Here's how the part is built. I have some questions about the finished solid (model axes, mm). A direction names the side the tool comes from. Coordinates: 2 decimals unless noted, no trailing zeros. Order: outer loops, then holes, each group sorted by start corner. A loop starts at its lowest first (then second) coordinate and runs counter-clockwise, first axis right, second up.
```python
from build123d import *

# Parameters (mm, degrees)
F0_W     = 7
F0_H     = 18
F2_DEPTH = 2
F3_DEPTH = 12.5
F4_R     = 0.6
F5_R     = 0.6
F6_R     = 2
F7_DEPTH = 25


with BuildPart() as f2:
    # F0 (on Front) → F2 (new body)
    with BuildSketch(Plane.XZ):
        Rectangle(F0_W, F0_H)
    extrude(amount=F2_DEPTH)

    # F1 (on face) → F3 (intersect, symmetric)
    with BuildSketch(Plane.XZ):
        with BuildLine():
            Line((-3.5, -9), (3.5, -9))
            Line((3.5, -9), (1.8, -2.5))
            Line((1.8, -2.5), (1.8, 2.5))
            ThreePointArc((1.8, 2.5), (0, 8.4978990818), (-1.8, 2.5))
            Line((-1.8, 2.5), (-1.8, -2.5))
            Line((-1.8, -2.5), (-3.5, -9))
        make_face()
    extrude(amount=F3_DEPTH, both=True, mode=Mode.INTERSECT)

    # F4
    f4_edges = [f2.edges().sort_by_distance(p)[0] for p in [
        (3.5, -1, -9),
    ]]
    fillet(f4_edges, radius=F4_R)

    # F5
    f5_edges = [f2.edges().sort_by_distance(p)[0] for p in [
        (-3.5, -1, -9),
    ]]
    fillet(f5_edges, radius=F5_R)

    # F6 (on face) → F7 (cut)
    with BuildSketch(Plane.XZ.offset(2)):
        with Locations((0, 5.2288549665)):
            Circle(F6_R)
    extrude(amount=-F7_DEPTH, mode=Mode.SUBTRACT)


solid = f2.part
```
Q1. For faces 4 (the flat face through (1.8, -1, 0)), 5 (the flat face through (-1.8, -1, 0)), 6 (the cylindrical face through (-0.434, -1.014, 3.276)), which set-ups out of +Z, -Z, +X, -X, +Y, -Y let a thin tool reach every point of the face, with its end or its side?
Q2. I need wall thicknesses on L1, parallel to Z at x = 0, y = -1.55; L2, parallel to X at y = -1.2, z = 5.25; L3, parallel to X at y = -0.6, z = 1.75. Which ranges of each line are inside material? Lowest first, please.
Q3. Will these pins go through, and if not, where does the flat tip stop? pin 1 (1 mm diameter, centred on y = -1.5, z = 0.5, fed in from -X); pin 2 (0.6 mm diameter, centred on y = -1.5, z = 0, fed in from +X); pin 3 (3 mm diameter, centred on x = 0, z = 5.23, fed in from +Y).
Q4. If we section it at A-A on x = 0: Write out the boundary of the cut face in (y, z).
Q5. If we section it at C-C on y = -1.2: Write out the boundary of the cut face in (x, z), then the cut area to 3 significant figures.
Q6. If we section it at D-D on z = 0.5: Write out the boundary of the cut face in (x, y).
Q7. If we section it at B-B on z = 4.75: Write out the boundary of the cut face in (x, y).
Q8. We'd pull the mould along Z, two halves only. Please class faces 1 (the flat face through (0, 0, 0)), 2 (the flat face through (0, -1, -9)), 3 (the flat face through (-2.54, -1.01, -5.33)): pulls with the +Z half, pulls with the -Z half, needs draft (parallel to the pull), parting line crosses it, or undercut.
Reply:
1. face 4: +X, +Y, -Y
1. face 5: -X, +Y, -Y
1. face 6: +Y, -Y
2. L1: z = -9 to 3.23, 7.23 to 8.5
2. L2: x = -3.27 to -2, 2 to 3.27
2. L3: x = -1.8 to 1.8
3. pin 1: stops at x = -1.8
3. pin 2: stops at x = 1.8
3. pin 3: passes through
4. outline: (-2, -9) - (0, -9) - (0, 3.23) - (-2, 3.23) - close; (-2, 7.23) - (0, 7.23) - (0, 8.5) - (-2, 8.5) - close
5. outline: (-3.3, -8.25) arc R0.6 ccw to (-2.72, -9) - (2.72, -9) arc R0.6 ccw to (3.3, -8.25) - (1.8, -2.5) - (1.8, 2.5) arc R3.27 ccw (long way) to (-1.8, 2.5) - (-1.8, -2.5) - close; hole circle Ø4 at (0, 5.23)
5. area: 71.9 mm2
6. outline: (-1.8, -2) - (1.8, -2) - (1.8, 0) - (-1.8, 0) - close
7. outline: (-3.23, -2) - (-1.94, -2) - (-1.94, 0) - (-3.23, 0) - close; (1.94, -2) - (3.23, -2) - (3.23, 0) - (1.94, 0) - close
8. face 1: needs draft
8. face 2: pulls with the -Z half
8. face 3: undercut
